```python
from build123d import *


with BuildPart() as part:
    # Sweep1: sweep along a path in Sketch2
    with BuildLine(Plane.XY) as sweep1_path:
        Line((0, 0), (0, 69))
        ThreePointArc((0, 69), (1.757359313, 73.242640687), (6, 75))
        Line((6, 75), (25, 75))
    # Sketch3 → Sweep1 (sweep)
    with BuildSketch(Plane(origin=(0, 0, 0), x_dir=(1, 0, 0), z_dir=(0, 1, 0))):
        Polygon((2, 2.309401077), (0, 1.154700538), (0, -1.154700538), (2, -2.309401077), (4, -1.154700538), (4, 1.154700538), align=None)
    sweep(path=sweep1_path.line)


solid = part.part
```
Part model, mm, in its own coordinate system. A direction names the side the tool comes from. Coordinates: 2 decimals unless noted, no trailing zeros. Loops run counter-clockwise (first coordinate to the right, second up) from the corner with the lowest first, then second, coordinate; pieces in that order, holes last. Notation, with made-up numbers: (13, -32.5) - (61, -32.5) arc R14 cw to (61, -9.5) - close; hole circle Ø3 at (39.25, -35). An arc over 180 degrees is marked (long way). Write item = value, one per line. Start each with the question number.
Item 1: Cut at B-B, the plane z = 0.3. Give the cut face in (x, y).
Item 2: 3-axis set-ups, long thin cutter, end or side, ignore diameter. For faces 1 (the flat face through (3.014, 34.983, -1.724)), 2 (the flat face through (16, 71, 0)), 3 (the flat face through (2.99, 34.98, 1.74)): which of +Z, -Z, +X, -X, +Y, -Y reach the whole face in a straight line?
Item 3: Wall check: L1, parallel to Y at x = 15, z = -1.15; L2, parallel to X at y = 37, z = 0.1; L3, parallel to X at y = 37, z = 1.25. Give the ranges that are in metal, low to high. Write a range as from..to.
Item 4: Cut at C-C, the plane x = 10.5. Give the cut face in (y, z), and give its area (3 significant figures).
Item 5: Flat gauge pins, fed straight in: pin 1 Ø1.8 at (x, z) = (19, -0.5) entering from -Y; pin 2 Ø1.8 at (y, z) = (21, -0.5) entering from +X. Where does each tip first touch, or does it go through?
Item 6: Cut at A-A, the plane y = 17.5. Give the cut face in (x, z), and give its area (3 significant figures).
The answers:
q1.outline = (0, 0) - (4, 0) - (4, 69) arc R2 cw to (6, 71) - (25, 71) - (25, 75) - (6, 75) arc R6 ccw to (0, 69) - close
q2.face_1 = -Z, +X, -Y
q2.face_2 = +Z, -Z, +X, -Y
q2.face_3 = +Z, +X, -Y
q3.L1 = 71..75
q3.L2 = 0..4
q3.L3 = 0.17..3.83
q4.outline = (71, -1.15) - (73, -2.31) - (75, -1.15) - (75, 1.15) - (73, 2.31) - (71, 1.15) - close
q4.area = 13.9 mm2
q5.pin_1 = 71
q5.pin_2 = 4
q6.outline = (0, -1.15) - (2, -2.31) - (4, -1.15) - (4, 1.15) - (2, 2.31) - (0, 1.15) - close
q6.area = 13.9 mm2
